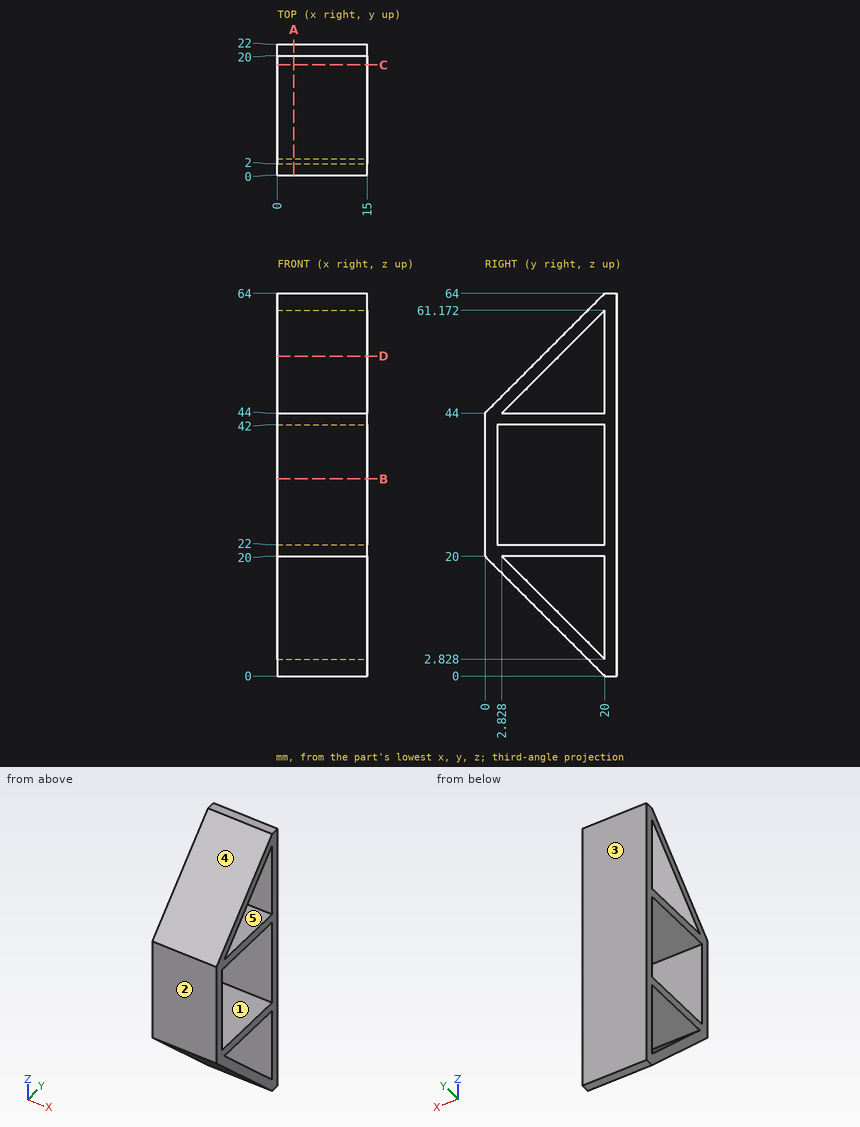
Study the drawing (mm; zero at the part's minimum x, y, z) and answer. A direction names the side the tool comes from. Give positions to 0.01 mm unless a question says otherwise; leave off trailing zeros. Loops run counter-clockwise (first coordinate to the right, second up) from the corner with the lowest first, then second, coordinate; pieces in that order, holes last. Notation, with made-up numbers: M -7.75,42 L 46.25,42 A9 ccw 46.25,52 Z; hole C 24.5,-37 d10. An arc over 180 degrees is marked long. One line per item, written item: value.
1. Section B-B on z = 33 is taken. Determine the outline of the cut face in (x, y).
Found:
outline: M 0,0 L 15,0 L 15,2 L 0,2 Z; M 0,20 L 15,20 L 15,22 L 0,22 Z
2. Find the intervals of material crossed by probe 1 along Y at (x, z) = (9.5, 34.5); probe 2 along Z at (x, y) = (7, 10.5); probe 3 along Z at (x, y) = (1.5, 13.75), in increasing order.
Found:
probe 1: 0 to 2, 20 to 22
probe 2: 9.5 to 12.33, 20 to 22, 42 to 44, 51.67 to 54.5
probe 3: 6.25 to 9.08, 20 to 22, 42 to 44, 54.92 to 57.75
3. Section D-D on z = 53.5 is taken. Determine the outline of the cut face in (x, y).
Found:
outline: M 0,9.5 L 15,9.5 L 15,12.33 L 0,12.33 Z; M 0,20 L 15,20 L 15,22 L 0,22 Z
4. Each of these flat-tipped pins is pushed along its axis until it touches: P1, Ø7.5, axis at x = 8, y = 13, coming from the +Z side; P2, Ø4.5, axis at x = 11, z = 8, coming from the -Y side; P3, Ø7.5, axis at x = 11, y = 12, coming from the -Z side; P4, Ø4, axis at y = 16.5, z = 24.5, coming from the +X side. Where does it stop, or does it pass through?
Found:
P1: z = 60.75
P2: y = 9.75
P3: z = 4.25
P4: through
5. For a pull along Y with two mould halves and no side action, classify the marked faces 3, 4 and 5 as pulls with the +Y half, pulls with the -Y half, needs draft (parallel to the pull), parting line crosses it, or undercut.
Found:
face 3: pulls with the +Y half
face 4: pulls with the -Y half
face 5: undercut
6. Section A-A on x = 2.75 is taken. Determine the outline of the cut face in (y, z).
Found:
outline: M 0,20 L 20,0 L 22,0 L 22,64 L 20,64 L 0,44 Z; hole M 2,22 L 20,22 L 20,42 L 2,42 Z; hole M 2.83,20 L 20,2.83 L 20,20 Z; hole M 2.83,44 L 20,44 L 20,61.17 Z
7. Section C-C on y = 18.5 is taken. Determine the outline of the cut face in (x, z).
Found:
outline: M 0,1.5 L 15,1.5 L 15,4.33 L 0,4.33 Z; M 0,20 L 15,20 L 15,22 L 0,22 Z; M 0,42 L 15,42 L 15,44 L 0,44 Z; M 0,59.67 L 15,59.67 L 15,62.5 L 0,62.5 Z
8. For the marked faces 1 and 2, determine the directions among +Z, -Z, +X, -X, +Y, -Y from which every point of the face is accessible in a straight line to the end or side of a thin tool.
Found:
face 1: +X, -X
face 2: +Z, -Z, +X, -X, -Y
